```python
from build123d import *

# Parameters (mm, degrees)
SKETCH1_R           = 1.7
BOSS_EXTRUDE1_DEPTH = 2
CHAMFER1_SIZE       = 1.5
CHAMFER2_SIZE       = 1.2
SKETCH2_W           = 22
SKETCH2_H           = 1.7
BOSS_EXTRUDE2_DEPTH = 1.1
SKETCH3_W           = 14
SKETCH3_H           = 7
SKETCH3_R           = 1.7
BOSS_EXTRUDE3_DEPTH = 1.1
BOSS_EXTRUDE4_DEPTH = 5.5
FILLET1_R           = 0.5
SKETCH5_W           = 6.1
SKETCH5_H           = 5.4
BOSS_EXTRUDE5_DEPTH = 4.3
SKETCH6_W           = 40.46
SKETCH6_H           = 5.4
CUT_EXTRUDE1_DEPTH  = 1.2
CUT_EXTRUDE2_DEPTH  = 2
SKETCH8_W           = 14
SKETCH8_H           = 5
CUT_EXTRUDE3_DEPTH  = 1


with BuildPart() as part:
    # Sketch1 → Boss-Extrude1 (new body)
    with BuildSketch(Plane(origin=(0, 0, 0), x_dir=(1, 0, 0), z_dir=(0, 1, 0))):
        Polygon((0, 0), (0, 9), (0.72, 9), (0.72, 27.6), (9.52, 27.6), (9.52, 29.7), (31.52, 29.7), (31.52, 27.6), (47.28, 27.6), (47.28, 9), (48, 9), (48, 0), align=None)
        with Locations(Location((19.42, 24.1, 0), (0, 0, 270))):
            Circle(SKETCH1_R, mode=Mode.SUBTRACT)
        with Locations(Location((6, 4.5, 0), (0, 0, 270))):
            Circle(SKETCH1_R, mode=Mode.SUBTRACT)
        with Locations(Location((42, 4.5, 0), (0, 0, 270))):
            Circle(SKETCH1_R, mode=Mode.SUBTRACT)
    extrude(amount=-BOSS_EXTRUDE1_DEPTH)

    # Chamfer1
    chamfer1_edges = [part.edges().sort_by_distance(p)[0] for p in [
        (5.12, 0, -27.6),
        (20.52, 0, -29.7),
        (39.4, 0, -27.6),
    ]]
    chamfer(chamfer1_edges, length=CHAMFER1_SIZE)

    # Chamfer2
    chamfer2_edges = [part.edges().sort_by_distance(p)[0] for p in [
        (19.42, 0, -25.8),
        (6, 0, -6.2),
        (42, 0, -6.2),
    ]]
    chamfer(chamfer2_edges, length=CHAMFER2_SIZE)

    # Sketch2 → Boss-Extrude2 (add)
    with BuildSketch(Plane.XZ.offset(2)):
        with Locations((20.52, -28.85)):
            Rectangle(SKETCH2_W, SKETCH2_H)
    extrude(amount=BOSS_EXTRUDE2_DEPTH)

    # Sketch3 → Boss-Extrude3 (add)
    with BuildSketch(Plane.XZ.offset(2)):
        with Locations((19.42, -24.5)):
            Rectangle(SKETCH3_W, SKETCH3_H)
        with Locations(Location((19.42, -24.1, 0), (0, 0, 90))):
            Circle(SKETCH3_R, mode=Mode.SUBTRACT)
    extrude(amount=BOSS_EXTRUDE3_DEPTH)

    # Sketch4 → Boss-Extrude4 (add)
    with BuildSketch(Plane.XZ.offset(2)):
        Polygon((0.72, -9.1), (47.28, -9.1), (47.28, -16.1), (44.08, -16.1), (44.08, -16.3), (44.08, -18.2), (42.26, -18.2), (42.26, -16), (38.56, -16), (38.56, -18.2), (35.18, -18.2), (35.18, -16), (31.48, -16), (31.48, -18.2), (30.28, -18.2), (30.28, -14.4), (26.6, -14.4), (26.6, -13.4), (11.4, -13.4), (11.4, -18.2), (10.02, -18.2), (10.02, -16), (6.32, -16), (6.32, -18.2), (3.72, -18.2), (3.72, -19.4), (0.72, -19.4), align=None)
    extrude(amount=BOSS_EXTRUDE4_DEPTH)

    # Fillet1
    fillet1_edges = [part.edges().sort_by_distance(p)[0] for p in [
        (6.32, -4.75, -18.2),
        (6.32, -4.75, -16),
        (10.02, -4.75, -16),
        (10.02, -4.75, -18.2),
        (31.48, -4.75, -18.2),
        (31.48, -4.75, -16),
        (35.18, -4.75, -16),
        (35.18, -4.75, -18.2),
        (38.56, -4.75, -18.2),
        (38.56, -4.75, -16),
        (42.26, -4.75, -16),
        (42.26, -4.75, -18.2),
    ]]
    fillet(fillet1_edges, radius=FILLET1_R)

    # Sketch5 → Boss-Extrude5 (add)
    with BuildSketch(Plane.XZ.offset(7.5)):
        with Locations((3.77, -11.8)):
            Rectangle(SKETCH5_W, SKETCH5_H)
    extrude(amount=BOSS_EXTRUDE5_DEPTH)

    # Sketch6 → Cut-Extrude1 (cut)
    with BuildSketch(Plane.XZ.offset(7.5)):
        with Locations((27.05, -11.8)):
            Rectangle(SKETCH6_W, SKETCH6_H)
    extrude(amount=-CUT_EXTRUDE1_DEPTH, mode=Mode.SUBTRACT)

    # Sketch7 → Cut-Extrude2 (cut)
    with BuildSketch(Plane.XZ.offset(6.3)):
        with BuildLine():
            Line((11.4, -13.4), (11.4, -13.12))
            ThreePointArc((11.4, -13.12), (11.60493511, -12.509074208), (12.14, -12.15))
            Line((12.14, -12.15), (14.52, -11.489318534))
            ThreePointArc((14.52, -11.489318534), (19.044112004, -10.644197545), (23.64, -10.4))
            Line((23.64, -10.4), (47.28, -10.4))
            Line((47.28, -10.4), (47.28, -14.5))
            Line((47.28, -14.5), (26.6, -14.5))
            Line((26.6, -14.5), (26.6, -13.4))
            Line((26.6, -13.4), (11.4, -13.4))
        make_face()
    extrude(amount=-CUT_EXTRUDE2_DEPTH, mode=Mode.SUBTRACT)

    # Sketch8 → Cut-Extrude3 (cut)
    with BuildSketch(Plane.XZ.offset(2)):
        with Locations((19.42, -18.5)):
            Rectangle(SKETCH8_W, SKETCH8_H)
    extrude(amount=-CUT_EXTRUDE3_DEPTH, mode=Mode.SUBTRACT)


solid = part.part
```
Part model, mm, in its own coordinate system. A direction names the side the tool comes from. Give positions to 0.01 mm unless a question says otherwise; leave off trailing zeros. Order: outer loops, then holes, each group sorted by start corner. A loop starts at its lowest first (then second) coordinate and runs counter-clockwise, first axis right, second up. Notation, with made-up numbers: M 30.25,20 L 75.25,20 A19 cw 75.25,54 Z; hole C -30,-27 d1. An arc over 180 degrees is marked long. Use a Markdown table: item, result. Add a question column.
(1) Mould opens along Z. For faces 4 (the face through (20, -3.1, -26)), 5 (the face through (9, -7, -14.5)), 6 (the face through (40, -5, -16)), 7 (the face through (26.6, -3, -14)) say: +Z half, -Z half, draft (parallel to the pull), parting line (faces both ways), or undercut.
(2) Probe line 1 along X through (y, z) = (-1.65, -4.5); line 2 along X through (y, z) = (-2.75, -14.5); line 3 along X through (y, z) = (-1.8, -24.1). List the from-to ranges inside material, lowest first. Write a range as [from, to].
(3) Drop flat-ended pins along their axis: P1, Ø1, axis at x = 30, y = -5, coming from the -Z side; P2, Ø0.9, axis at y = -1.5, z = -28, coming from the +X side; P3, Ø1.2, axis at x = 11.5, y = -2.5, coming from the +Z side; P4, Ø1, axis at x = 18, y = -5.5, coming from the -Z side. Give the stop position or say it passes through.
(4) Saw through at D-D, the plane x = 13. Give the cut face in (y, z).
(5) Saw through at C-C, the plane y = -2.5. Give the number of separate pieces and of enclosed holes in the cut face, and give its area (3 significant figures).
(6) Saw through at A-A, the plane z = -4.5. Give the cut face in (x, y), and give its area (3 significant figures).
(7) 3-axis set-ups, long thin cutter, end or side, ignore diameter. For faces 1 (the face through (0.72, -5, -14)), 2 (the face through (31.52, -1.5, -28.3)), 3 (the face through (44.08, -5, -17)): which of +Z, -Z, +X, -X, +Y, -Y reach the whole face in a straight line?
(8) Saw through at B-B, the plane z = -24.1. Give the cut face in (x, y).
Answer key:
| question | item | result |
|---|---|---|
| 1 | face 4 | draft |
| 1 | face 5 | +Z half |
| 1 | face 6 | -Z half |
| 1 | face 7 | undercut |
| 2 | line 1 | [0, 4.3], [7.7, 40.3], [43.7, 48] |
| 2 | line 2 | [0.72, 11.4], [30.28, 47.28] |
| 2 | line 3 | [0.72, 17.72], [21.12, 47.28] |
| 3 | P1 | z = -18.2 |
| 3 | P2 | x = 47.28 |
| 3 | P3 | z = 0 |
| 3 | P4 | z = -10.86 |
| 4 | outline | M -6.3,-11.91 L -4.3,-11.91 L -4.3,-13.4 L -2,-13.4 L -2,-16 L -1,-16 L -1,-21 L -3.1,-21 L -3.1,-29.7 L -1.5,-29.7 L 0,-28.2 L 0,0 L -2,0 L -2,-9.1 L -6.3,-9.1 Z |
| 5 | separate pieces | 2 |
| 5 | enclosed holes | 1 |
| 5 | area | 436 mm^2 |
| 6 | outline | M 0,-2 L 4.3,-2 L 4.3,-1.2 L 3.1,0 L 0,0 Z; M 7.7,-2 L 40.3,-2 L 40.3,-1.2 L 39.1,0 L 8.9,0 L 7.7,-1.2 Z; M 43.7,-2 L 48,-2 L 48,0 L 44.9,0 L 43.7,-1.2 Z |
| 6 | area | 79.5 mm^2 |
| 7 | face 1 | -Z, -X, +Y, -Y |
| 7 | face 2 | -Z, +X, +Y |
| 7 | face 3 | -Z, +X, -Y |
| 8 | outline | M 0.72,-2 L 12.42,-2 L 12.42,-3.1 L 17.72,-3.1 L 17.72,-1.2 L 16.52,0 L 0.72,0 Z; M 21.12,-3.1 L 26.42,-3.1 L 26.42,-2 L 47.28,-2 L 47.28,0 L 22.32,0 L 21.12,-1.2 Z |
